```python
from build123d import *

# Parameters (mm, degrees)
F0_W     = 434.34
F0_H     = 254
F1_DEPTH = 558.8
F2_R     = 88.136421
F3_DEPTH = 76.2


with BuildPart() as f1:
    # F0 (on Top) → F1 (new body)
    with BuildSketch(Plane.XY):
        Rectangle(F0_W, F0_H)
    extrude(amount=F1_DEPTH)

    # F2 (on face) → F3 (join)
    with BuildSketch(Plane.XY.offset(558.8)):
        Circle(F2_R)
    extrude(amount=F3_DEPTH)

    # F4 (on Front) → F5 (revolve)
    with BuildSketch(Plane.XZ):
        Polygon((-109.097786, 588.431537), (0, 588.431537), (0, 725.384057), (0, 843.766749), (0, 1038.749933), (0, 1161.775112), (0, 1570.658565), (-109.097786, 1570.658565), (-109.097786, 1455.510974), (-81.243046, 1455.510974), (-81.243046, 1440.529093), (-118.768431, 1403.003693), (-127.059057, 1403.003693), (-127.059057, 1314.976215), (-118.382715, 1314.976215), (-81.243046, 1277.836561), (-81.243046, 1161.775112), (-109.097786, 1161.775112), (-109.097786, 1038.749933), (-81.243046, 1038.749933), (-81.243046, 973.755538), (-102.134109, 973.755538), (-102.134109, 843.766749), (-81.243046, 843.766749), (-81.243046, 725.384057), (-109.097786, 725.384057), align=None)
    revolve(axis=Axis((0, 0, 1635.457158), (0, 0, 1)))


solid = f1.part
```
The model under review builds one solid part; all positions refer to its coordinate system, in mm. A direction names the side the tool comes from. Give positions to 0.01 mm unless a question says otherwise; leave off trailing zeros. Write each loop counter-clockwise with the first axis right and the second up, starting at its lowest first coordinate (ties: lowest second). Pieces come first, ordered by that corner, then holes.
(1) To check wall thickness, follow L1, parallel to Z at x = -10.5, y = 94; L2, parallel to Z at x = -122, y = 53; L3, parallel to Y at x = 60, z = 424. State the ranges of each line that lie inside material, in increasing order.
(2) Consider section A-A, the plane z = 944.5. Give the boundary of the cut face in (x, y), and give its area (3 significant figures).
(3) The part is to be moulded in two halves that separate along Z. For faces 4 (the flat face through (-2, -2, 1570.659)), 5 (the conical face through (18.121, 81.603, 1438.182)), 6 (the flat face through (-3, -127, 275)), say which applies: released by +Z, released by -Z, zero draft, split by the parting line, or undercut.
(4) Consider section B-B, the plane z = 1259. Give the boundary of the cut face in (x, y), and give its area (3 significant figures).
(5) For P1, Ø4, axis at y = -28, z = 1124, coming from the +X side; P2, Ø10, axis at y = 19, z = 866.5, coming from the +X side; P3, Ø12, axis at x = 49, z = 292.5, coming from the -Y side, all flat-tipped, find the tip position at first contact; note any pin that passes through.
(6) Tool access review of faces 1 (the flat face through (-217.17, -2, 275)), 2 (the flat face through (69, 45, 843.767)), 3 (the cylindrical face through (16.541, -125.978, 1358.374)): name each direction out of +Z, -Z, +X, -X, +Y, -Y from which nothing blocks a thin tool from reaching the whole face with its end or side.
Returned:
1. L1: z = 0 to 558.8, 588.43 to 725.38, 843.77 to 973.76, 1038.75 to 1161.78, 1291.18 to 1427.19, 1455.51 to 1570.66
1. L2: z = 0 to 558.8
1. L3: y = -127 to 127
2. outline: circle Ø204.27 at (0, 0)
2. area: 32,800 mm2
3. face 4: released by +Z
3. face 5: undercut
3. face 6: zero draft
4. outline: circle Ø162.49 at (0, 0)
4. area: 20,700 mm2
5. P1: stops at x = 105.95
5. P2: stops at x = 101.17
5. P3: stops at y = -127
6. face 1: +Z, -Z, -X, +Y, -Y
6. face 2: none
6. face 3: +Z
